Could you check a few things on this drawing? It's one solid part, dimensions in mm from its lowest x, y, z. Round coordinates to 2 decimals unless told otherwise and drop trailing zeros. Write each loop counter-clockwise with the first axis right and the second up, starting at its lowest first coordinate (ties: lowest second). Pieces come first, ordered by that corner, then holes. Notation, with made-up numbers: (-21.75, 2.25) -> (3.25, 2.25) arc R21 cw to (3.25, 32.25) -> close; hole circle Ø11 at (-30.75, 73). An arc over 180 degrees is marked (long way). Put each result on its own line as item: value. Start each with the question number.
1) I want a section at B-B, the plane x = 44. List the corners of the cut face in (y, z) for me.
2) We'd pull the mould along X, two halves only. Please class the marked faces 1 and 2: released by +X, released by -X, zero draft, split by the parting line, or undercut.
3) I want a section at C-C, the plane y = 48. List the corners of the cut face in (x, z) for me, then the cut area to 3 significant figures.
4) Will these pins go through, and if not, where does the flat tip stop? P1, Ø5, axis at x = 36.5, y = 49, coming from the +Z side; P2, Ø0.8, axis at x = 120.5, z = 2.5, coming from the +Y side; P3, Ø5.5, axis at x = 93.5, z = 7.5, coming from the +Y side.
5) I want a section at A-A, the plane y = 100. List the corners of the cut face in (x, z) for me.
6) I want a section at D-D, the plane z = 7.5. List the corners of the cut face in (x, y) for me, then the cut area to 3 significant figures.
7) If I drill on line 1 along Y through (x, z) = (146, 7); line 2 along X through (y, z) = (96.5, 4.5); line 3 along X through (y, z) = (91, 5.5), over which ranges is the centre line in solid material (lowest first)? Write a range as [from, to].
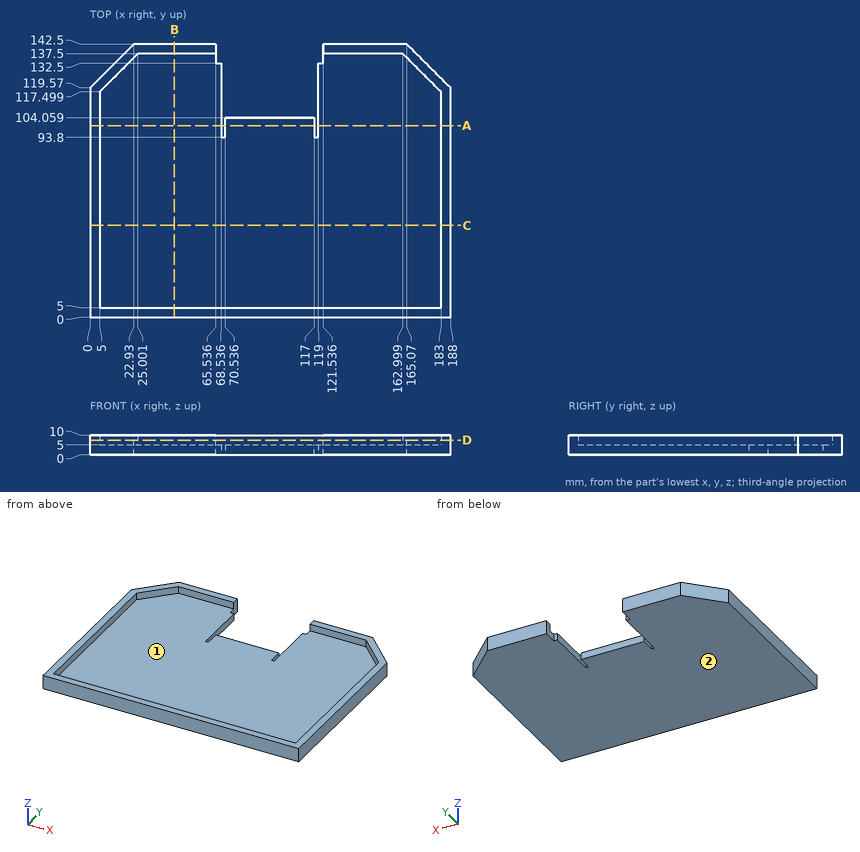
Findings:
1. outline: (0, 0) -> (142.5, 0) -> (142.5, 10) -> (137.5, 10) -> (137.5, 5) -> (5, 5) -> (5, 10) -> (0, 10) -> close
2. face 1: undercut
2. face 2: zero draft
3. outline: (0, 0) -> (188, 0) -> (188, 10) -> (183, 10) -> (183, 5) -> (5, 5) -> (5, 10) -> (0, 10) -> close
3. area: 990 mm2
4. P1: stops at z = 5
4. P2: stops at y = 132.5
4. P3: stops at y = 104.06
5. outline: (0, 0) -> (68.54, 0) -> (68.54, 5) -> (5, 5) -> (5, 10) -> (0, 10) -> close; (70.54, 0) -> (117, 0) -> (117, 5) -> (70.54, 5) -> close; (119, 0) -> (188, 0) -> (188, 10) -> (183, 10) -> (183, 5) -> (119, 5) -> close
6. outline: (0, 0) -> (188, 0) -> (188, 119.57) -> (165.07, 142.5) -> (121.54, 142.5) -> (121.54, 137.5) -> (163, 137.5) -> (183, 117.5) -> (183, 5) -> (5, 5) -> (5, 117.5) -> (25, 137.5) -> (65.54, 137.5) -> (65.54, 142.5) -> (22.93, 142.5) -> (0, 119.57) -> close
6. area: 2,800 mm2
7. line 1: y = [0, 5], [137.5, 142.5]
7. line 2: x = [0, 68.54], [70.54, 117], [119, 188]
7. line 3: x = [0, 5], [183, 188]
